from build123d import *

# Parameters (mm, degrees)
F0_W     = 42
F0_H     = 45
F1_DEPTH = 5
F2_R     = 5
F3_DEPTH = 7.4
F4_W     = 42
F4_H     = 10
F5_DEPTH = 7.5
F7_DEPTH = 42
F9_DEPTH = 42


with BuildPart() as f1:
    # F0 (on Top) → F1 (new body)
    with BuildSketch(Plane.XY):
        Rectangle(F0_W, F0_H)
    extrude(amount=F1_DEPTH)

    # F2 (on face) → F3 (join)
    with BuildSketch(Plane.XY.offset(5)):
        with Locations((-13.378, 0)):
            Circle(F2_R)
        with Locations((13.378, 0)):
            Circle(F2_R)
    extrude(amount=F3_DEPTH)

    # F4 (on face) → F5 (join)
    with BuildSketch(Plane.XY.offset(5)):
        with Locations((0, 17.5)):
            Rectangle(F4_W, F4_H)
        with Locations((0, -17.5)):
            Rectangle(F4_W, F4_H)
    extrude(amount=F5_DEPTH)

    # F6 (on face) → F7 (join)
    with BuildSketch(Plane.YZ.offset(21)):
        Polygon((22.5, 12.5), (22.5, 0), (35, 12.5), align=None)
    extrude(amount=-F7_DEPTH)

    # F8 (on face) → F9 (join)
    with BuildSketch(Plane.YZ.offset(21)):
        Polygon((-35, 12.5), (-22.5, 0), (-22.5, 12.5), align=None)
    extrude(amount=-F9_DEPTH)


solid = f1.part
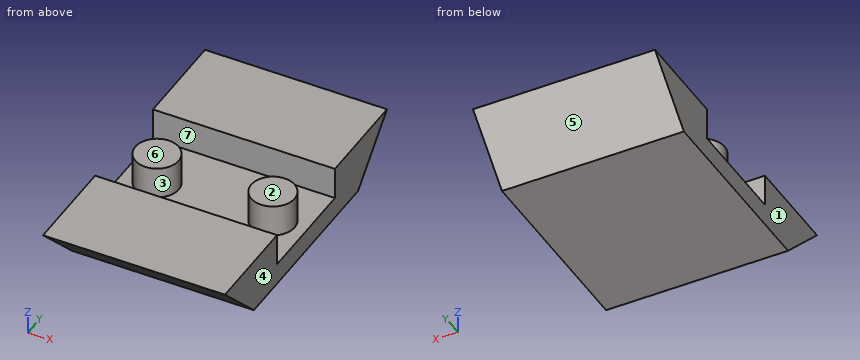
Verification items for the finished model (mm, model axes). Face numbers are marked on the shaded views. A direction names the side the tool comes from. Coordinates: 2 decimals unless noted, no trailing zeros. Order: outer loops, then holes, each group sorted by start corner. A loop starts at its lowest first (then second) coordinate and runs counter-clockwise, first axis right, second up. Notation, with made-up numbers: M -12,-2 L 40,-2 A21 ccw 40,3 Z; hole C 7.5,7.5 d11. An arc over 180 degrees is marked long. One line per item, written item: value. Start each with the question number.
Item 1: Thickness scan on probe 1 along Y at (x, z) = (-14.5, 5.5); probe 2 along Y at (x, z) = (15.5, 11.5); probe 3 along Z at (x, y) = (-15.5, 6.5). Record the ranges inside material, lowest first.
Item 2: Sectioned sample at A-A on y = 0. Record the cut outline in (x, z).
Item 3: Sectioned sample at C-C on x = 1. Record the cut outline in (y, z).
Item 4: Depth check by flat-ended pin: P1, Ø4, axis at x = 7, z = 10, coming from the +Y side; P2, Ø4, axis at x = -5.5, z = 7.5, coming from the -Y side; P3, Ø7.5, axis at x = 7.5, y = 5, coming from the +Z side. Enter the tip coordinate at first touch or a pass-through.
Item 5: Sectioned sample at B-B on z = 8. Record the cut outline in (x, y), then the cut area to 3 significant figures.
Item 6: Access from +Z, -Z, +X, -X, +Y, -Y to the whole of each face (thin tool, end or side, straight path). Record for the marked faces 1, 2 and 3.
Item 7: Mould release check, pull along Y, two halves, no side actions. Record for the marked faces 4, 5, 6 and 7: pulls with the +Y half, pulls with the -Y half, needs draft (parallel to the pull), parting line crosses it, or undercut.
Item 8: Sectioned sample at D-D on z = 2.75. Record the cut outline in (x, y).
Calculated:
1. probe 1: -28 to -12.5, -4.87 to 4.87, 12.5 to 28
1. probe 2: -34 to -12.5, -4.53 to 4.53, 12.5 to 34
1. probe 3: 0 to 5
2. outline: M -21,0 L 21,0 L 21,5 L 18.38,5 L 18.38,12.4 L 8.38,12.4 L 8.38,5 L -8.38,5 L -8.38,12.4 L -18.38,12.4 L -18.38,5 L -21,5 Z
3. outline: M -35,12.5 L -22.5,0 L 22.5,0 L 35,12.5 L 12.5,12.5 L 12.5,5 L -12.5,5 L -12.5,12.5 Z
4. P1: y = 34.5
4. P2: y = -32
4. P3: z = 12.4
5. outline: M -21,-30.5 L 21,-30.5 L 21,-12.5 L -21,-12.5 Z; M -21,12.5 L 21,12.5 L 21,30.5 L -21,30.5 Z; C -13.38,0 d10; C 13.38,0 d10
5. area: 1,670 mm^2
6. face 1: +Z, -Z, -X, +Y, -Y
6. face 2: +Z, +X, -X
6. face 3: +Z
7. face 4: needs draft
7. face 5: pulls with the +Y half
7. face 6: undercut
7. face 7: undercut
8. outline: M -21,-25.25 L 21,-25.25 L 21,25.25 L -21,25.25 Z
